Geometry: final body of the model. Coordinates: model frame, mm. Round coordinates to 2 decimals unless told otherwise and drop trailing zeros. Order: outer loops, then holes, each group sorted by start corner. A loop starts at its lowest first (then second) coordinate and runs counter-clockwise, first axis right, second up. Notation, with made-up numbers: M 54.5,42.5 L 101.5,42.5 A35 ccw 101.5,79.5 Z; hole C -25.75,-12 d1. An arc over 180 degrees is marked long. Return JSON: item names as keys, results as strings. Group by question number.
Q1. Cut plane D-D on x = 55. Output: boundary loops of the cut face in (y, z) (3 decimals), and give its area (3 significant figures).
Q2. Cut plane B-B on x = -41. Output: boundary loops of the cut face in (y, z).
Q3. Cut plane C-C on y = 0.65. Count the separate pieces of the cut face and the enclosed holes in it, and give its area (3 significant figures).
Q4. Ray query, probe 1 along X at (y, z) = (1, 30.5); probe 2 along Z at (x, y) = (-19, 0.5); probe 3 along Z at (x, y) = (-55, 0.8) (3 decimals). Return the intervals inside material, ascending.
Q5. Cut plane A-A on z = 2. Output: boundary loops of the cut face in (x, y), and give its area (3 significant figures).
```python
from build123d import *

# Parameters (mm, degrees)
SKIZZE1_W                             = 172
SKIZZE1_H                             = 185
AUFSATZ_LINEAR_AUSTRAGEN1_DEPTH       = 2
DURCHGANGSLOCH_F_R_M31_D              = 3.4
F_3_8_3_8_DURCHMESSER_BOHRUNG1_D      = 3.8
F_3_8_3_8_DURCHMESSER_BOHRUNG1_DEPTH  = 10
F_3_8_3_8_DURCHMESSER_BOHRUNG1_TIP    = 1.141635176
F_3_4_3_4_DURCHMESSER_LANGLOCH1_DEPTH = 2
SKIZZE5_W                             = 20
SKIZZE5_H                             = 75
SKIZZE5_W_2                           = 60
SKIZZE5_H_2                           = 55
SCHNITT_LINEAR_AUSTRAGEN1_DEPTH       = 10
F_4_3_4_79_DURCHMESSER_BOHRUNG1_D     = 4.79
DURCHGANGSLOCH_F_R_M32_D              = 3.4
M3X0_5_GEWINDEBOHRUNG2_D              = 2.5
M3X0_5_GEWINDEBOHRUNG3_D              = 2.5
VERRUNDUNG1_R                         = 1
M2X0_4_GEWINDEBOHRUNG1_D              = 1.6


# Read off the part's stored shape, not the designer's step: Ø3.4 (3.4) Durchmesser Langloch1
with BuildPart() as part:
    # Skizze1 → Aufsatz-Linear austragen1 (new body)
    with BuildSketch(Plane(origin=(0, 0, 0), x_dir=(1, 0, 0), z_dir=(0, 1, 0))):
        Rectangle(SKIZZE1_W, SKIZZE1_H)
    extrude(amount=AUFSATZ_LINEAR_AUSTRAGEN1_DEPTH)

    # Durchgangsloch für M31 (through all)
    with Locations(Plane(origin=(0, 2, 0), x_dir=(1, 0, 0), z_dir=(0, 1, 0))):
        with Locations((81.5, -57.5)):
            Hole(DURCHGANGSLOCH_F_R_M31_D / 2)

    # Ø3.8 (3.8) Durchmesser Bohrung1
    with Locations(Plane(origin=(0, 2, 0), x_dir=(1, 0, 0), z_dir=(0, 1, 0))):
        with Locations((-81.5, -57.5), (-81.5, 57.5)):
            Hole(F_3_8_3_8_DURCHMESSER_BOHRUNG1_D / 2, depth=F_3_8_3_8_DURCHMESSER_BOHRUNG1_DEPTH)
            with Locations((0, 0, -(F_3_8_3_8_DURCHMESSER_BOHRUNG1_DEPTH + F_3_8_3_8_DURCHMESSER_BOHRUNG1_TIP / 2))):  # 118° drill point
                Cone(0, F_3_8_3_8_DURCHMESSER_BOHRUNG1_D / 2, F_3_8_3_8_DURCHMESSER_BOHRUNG1_TIP, mode=Mode.SUBTRACT)

    # Ø3.4 (3.4) Durchmesser Langloch1 outline → Ø3.4 (3.4) Durchmesser Langloch1 (cut)
    with BuildSketch(Plane(origin=(0, 0, 0), x_dir=(1, 0, 0), z_dir=(0, 1, 0))):
        with BuildLine():
            Line((79.8, 57.8), (79.8, 57.2))
            ThreePointArc((79.8, 57.2), (81.5, 55.5), (83.2, 57.2))
            Line((83.2, 57.2), (83.2, 57.8))
            ThreePointArc((83.2, 57.8), (81.5, 59.5), (79.8, 57.8))
        make_face()
    extrude(amount=F_3_4_3_4_DURCHMESSER_LANGLOCH1_DEPTH, mode=Mode.SUBTRACT)

    # Skizze5 → Schnitt-Linear austragen1 (cut)
    with BuildSketch(Plane(origin=(0, 0, 0), x_dir=(1, 0, 0), z_dir=(0, 1, 0))):
        with Locations((26, -15)):
            Rectangle(SKIZZE5_W, SKIZZE5_H)
        with Locations((-46, -25)):
            Rectangle(SKIZZE5_W_2, SKIZZE5_H_2)
    extrude(amount=SCHNITT_LINEAR_AUSTRAGEN1_DEPTH, mode=Mode.SUBTRACT)

    # Ø4.3 (4.79) Durchmesser Bohrung1 (through all)
    with Locations(Plane(origin=(0, 2, 0), x_dir=(1, 0, 0), z_dir=(0, 1, 0))):
        with Locations((-55, -73.5), (55, -73.5)):
            Hole(F_4_3_4_79_DURCHMESSER_BOHRUNG1_D / 2)

    # Durchgangsloch für M32 (through all)
    with Locations(Plane(origin=(0, 2, 0), x_dir=(1, 0, 0), z_dir=(0, 1, 0))):
        with Locations((46, -21.5), (76, -21.5)):
            Hole(DURCHGANGSLOCH_F_R_M32_D / 2)

    # M3x0.5 Gewindebohrung2 (through all)
    with Locations(Plane(origin=(0, 2, 0), x_dir=(1, 0, 0), z_dir=(0, 1, 0))):
        with Locations((-68, 27.5), (-19, 85.5), (-68, 85.5), (-19, 27.5), (-0.6, 29.1), (-82, 88.5), (-0.6, 88.5), (-82, 29.1)):
            Hole(M3X0_5_GEWINDEBOHRUNG2_D / 2)

    # M3x0.5 Gewindebohrung3 (through all)
    with Locations(Plane(origin=(0, 2, 0), x_dir=(1, 0, 0), z_dir=(0, 1, 0))):
        with Locations((22.5, 27.5), (81.5, 89.5), (22.5, 89.5), (81.5, 27.5), (22.5, 39.5)):
            Hole(M3X0_5_GEWINDEBOHRUNG3_D / 2)

    # Verrundung1
    verrundung1_edges = [part.edges().sort_by_distance(p)[0] for p in [
        (16, 1, -22.5),
        (16, 1, 52.5),
        (36, 1, 52.5),
        (36, 1, -22.5),
        (-76, 1, -2.5),
        (-76, 1, 52.5),
        (-16, 1, 52.5),
        (-16, 1, -2.5),
        (-86, 1, -92.5),
        (86, 1, -92.5),
        (86, 1, 92.5),
        (-86, 1, 92.5),
    ]]
    fillet(verrundung1_edges, radius=VERRUNDUNG1_R)

    # M2x0.4 Gewindebohrung1 (through all)
    with Locations(Plane(origin=(0, 2, 0), x_dir=(1, 0, 0), z_dir=(0, 1, 0))):
        with Locations((10.795, -12.62), (-10.795, -12.62), (-10.795, 2.62), (10.795, 2.62), (40.205, 70.62), (40.205, 55.38), (59.795, 55.38), (59.795, 70.62)):
            Hole(M2X0_4_GEWINDEBOHRUNG1_D / 2)


solid = part.part
```
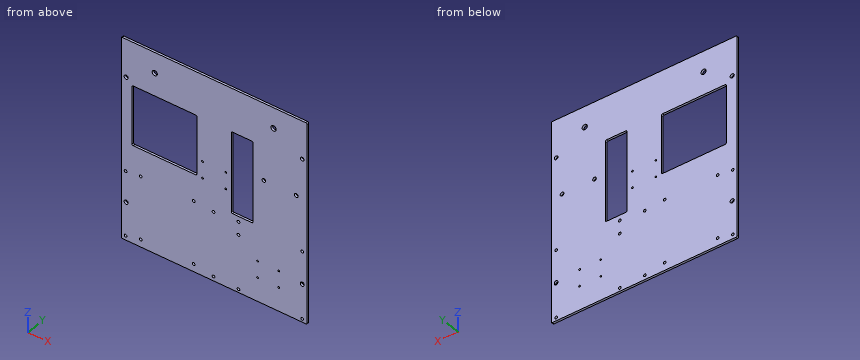
Result sheet:
{
 "1": {"outline": "M 0,-92.5 L 2,-92.5 L 2,71.105 L 0,71.105 Z; M 0,75.895 L 2,75.895 L 2,92.5 L 0,92.5 Z", "area": "360 mm²"},
 "2": {"outline": "M 0,-92.5 L 2,-92.5 L 2,-2.5 L 0,-2.5 Z; M 0,52.5 L 2,52.5 L 2,92.5 L 0,92.5 Z"},
 "3": {"separate pieces": "1", "enclosed holes": "31", "area": "26,800 mm²"},
 "4": {"probe 1": "x = -86 to -76, -16 to 16, 36 to 86", "probe 2": "z = -92.5 to -86.75, -84.25 to -28.75, -26.25 to -2.5, 52.5 to 92.5", "probe 3": "z = -92.5 to -2.5, 52.5 to 71.105, 75.895 to 92.5"},
 "5": {"outline": "M -86,0 L -76,0 L -76,2 L -86,2 Z; M -16,0 L 16,0 L 16,2 L -16,2 Z; M 36,0 L 86,0 L 86,2 L 36,2 Z", "area": "184 mm²"}
}
